The listing builds one solid part. Answer for the finished solid, in the listing's coordinates (mm). Face numbers are marked on the shaded views. A direction names the side the tool comes from. Coordinates: 2 decimals unless noted, no trailing zeros. Order: outer loops, then holes, each group sorted by start corner. A loop starts at its lowest first (then second) coordinate and runs counter-clockwise, first axis right, second up. Notation, with made-up numbers: (-18.5, 22.25) -> (35.5, 22.25) arc R24 cw to (35.5, 61.25) -> close; hole circle Ø3 at (73, 64). An arc over 180 degrees is marked (long way). Return JSON: item names as keys, results as strings.
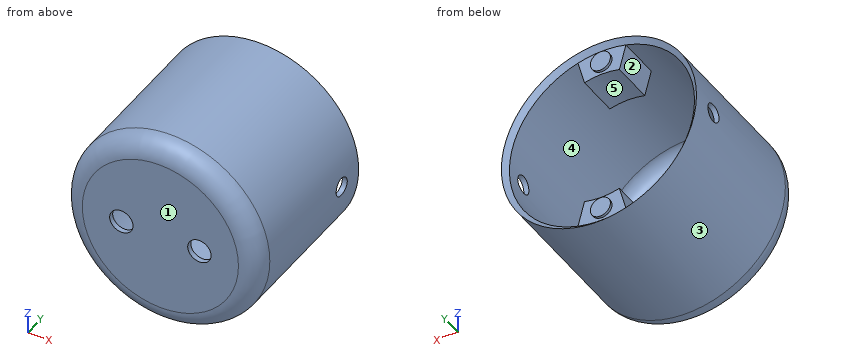
Autodesk Inventor part; units mm, degrees
ref_plane "Plano de trabajo1" through (-8, 0, 0) normal (1, 0, 0) x (0, 1, 0)
ref_plane "XZ Plane" through (0, 0, 0) normal (0, 1, 0) x (-1, 0, 0)
ref_plane "XY Plane" through (0, 0, 0) normal (0, 0, 1) x (1, 0, 0)
sketch "Boceto1" plane through (0, 0, 0) normal (0, 0, 1) x (1, 0, 0)
  line L0 (0, 0) -> (-4.6715, 0)
  line L1 (-5.8393, 9.9269) -> (-5.8393, 1.1679)
  line L2 (-5.5393, 9.6269) -> (-5.5393, 1.1679)
  arc A0 (-5.8393, 1.1679) -> (-4.6715, 0) centre (-4.6715, 1.1679) ccw
  arc A1 (-5.5393, 1.1679) -> (-4.6715, 0.3) centre (-4.6715, 1.1679) ccw
  line L3 (0, 0) -> (-4.6715, 0)
  line L4 (0, 0.3) -> (-4.6715, 0.3)
  line L5 (0, 0.3) -> (0, 0)
  line L6 (-5.8393, 9.9269) -> (-5.5393, 9.6269)
revolve "Revolución1" add sketch "Boceto1" angle 360 about axis through (0, 0.3, 0) along (0, -1, 0)
sketch "Boceto2" plane through (0, 0, 0) normal (1, 0, 0) x (0, 1, 0)
  line L0 (9.6269, 5.5393) -> (1.1679, 5.5393)
  line L1 (9.6269, -5.5393) -> (1.1679, -5.5393)
  line L2 (9.6269, 5.5393) -> (9.6269, 4.0393)
  line L3 (9.6269, -5.5393) -> (9.6269, 5.5393)
  line L4 (9.6269, 4.0393) -> (7.1269, 4.0393)
  line L5 (7.1269, 4.0393) -> (7.1269, 5.5393)
  line L6 (9.6269, 5.5393) -> (7.1269, 5.5393)
  line L7 (9.6269, 0) -> (13.8106, 0)
  line L8 (9.6269, -5.5393) -> (9.6269, -4.0393)
  line L9 (9.6269, -4.0393) -> (7.1269, -4.0393)
  line L10 (7.1269, -4.0393) -> (7.1269, -5.5393)
  point P0 (0, 0)
  dimension "d1" = 1.5
  dimension "d2" = 2.5
  dimension "d3" = 1.5
  dimension "d4" = 2.5
revolve "Revolución2" add sketch "Boceto2" angle 30 mid plane about axis through (0, 9.6269, 0) along (0, 1, 0)
sketch "Boceto3" plane through (0, 9.6269, 0) normal (0, 1, 0) x (1, 0, 0)
  line L0 (-1.0455, -3.9017) -> (-1.4337, -5.3506)
  arc A0 (-1.4337, -5.3506) -> (1.4337, -5.3506) centre (0, 0) ccw
  line L1 (1.0455, -3.9017) -> (1.4337, -5.3506)
  arc A1 (-1.0455, -3.9017) -> (1.0455, -3.9017) centre (0, 0) ccw
  line L2 (1.4337, 5.3506) -> (1.0455, 3.9017)
  arc A2 (1.4337, 5.3506) -> (-1.4337, 5.3506) centre (0, 0) ccw
  line L3 (-1.0455, 3.9017) -> (-1.4337, 5.3506)
  arc A3 (1.0455, 3.9017) -> (-1.0455, 3.9017) centre (0, 0) ccw
  circle A4 centre (0, 4.7895) radius 0.6
  circle A5 centre (0, -4.7895) radius 0.6
  dimension "d9" = 1.2
  dimension "d10" = 1.2
extrude "Extrusión1" add sketch "Boceto3" along normal blind 0.155 contours A4 | A5
ref_plane "Plano de trabajo1" through (-8, 0, 0) normal (1, 0, 0) x (0, 1, 0)
sketch "Boceto6" plane through (-8, 0, 0) normal (1, 0, 0) x (0, 1, 0)
  line L0 (1.1679, -5.8393) -> (1.1679, 5.8393)
  line L1 (9.9269, -5.8393) -> (9.9269, 5.8393)
  line L2 (0, -4.6715) -> (0, 4.6715)
  line L3 (1.1679, -5.8393) -> (1.1679, 5.8393)
  circle A0 centre (8.2551, 0) radius 0.55
  point P0 (0, 0)
extrude "Extrusión2" cut sketch "Boceto6" along normal blind 16
sketch "Boceto7" plane through (0, 0, 0) normal (0, -1, 0) x (1, 0, 0)
  circle A0 centre (-2.3358, 0) radius 0.7
  circle A1 centre (2.3358, 0) radius 0.7
  point P0 (0, 0)
  dimension "d17" = 1.4
  dimension "d18" = 1.4
extrude "Extrusión3" cut sketch "Boceto7" against normal blind 3
properties part number "cuerpo"
Item 1: The part is cut by section A-A on z = 0. Determine the outline of the cut face in (x, y).
Answer list:
{"outline": "(-5.84, 1.17) arc R1.17 ccw to (-4.67, 0) -> (-3.04, 0) -> (-3.04, 0.3) -> (-4.67, 0.3) arc R0.87 cw to (-5.54, 1.17) -> (-5.54, 7.71) -> (-5.84, 7.71) -> close; (-5.84, 8.81) -> (-5.54, 8.81) -> (-5.54, 9.63) -> (-5.84, 9.93) -> close; (-1.64, 0) -> (1.64, 0) -> (1.64, 0.3) -> (-1.64, 0.3) -> close; (3.04, 0) -> (4.67, 0) arc R1.17 ccw to (5.84, 1.17) -> (5.84, 7.71) -> (5.54, 7.71) -> (5.54, 1.17) arc R0.87 cw to (4.67, 0.3) -> (3.04, 0.3) -> close; (5.54, 8.81) -> (5.84, 8.81) -> (5.84, 9.93) -> (5.54, 9.63) -> close"}
Item 2: Find the intervals of material crossed by probe 1 along X at (y, z) = (8, 4.25); probe 2 along Y at (x, z) = (1.25, 1.25); probe 3 along X at (y, z) = (8.25, -3), in increasing order.
Answer list:
{"probe 1": "-4 to -3.55, -1.14 to 1.14, 3.55 to 4", "probe 2": "0 to 0.3", "probe 3": "-5.01 to -4.66, 4.66 to 5.01"}
Item 3: The part is cut by section B-B on y = 4.75. Determine the outline of the cut face in (x, z).
Answer list:
{"outline": "circle Ø11.68 at (0, 0); hole circle Ø11.08 at (0, 0)"}
Item 4: The part is cut by section C-C on x = 0. Determine the outline of the cut face in (y, z).
Answer list:
{"outline": "(0, -4.67) arc R1.17 ccw to (1.17, -5.84) -> (9.93, -5.84) -> (9.63, -5.54) -> (9.63, -5.39) -> (9.78, -5.39) -> (9.78, -4.19) -> (9.63, -4.19) -> (9.63, -4.04) -> (7.13, -4.04) -> (7.13, -5.54) -> (1.17, -5.54) arc R0.87 cw to (0.3, -4.67) -> (0.3, 4.67) arc R0.87 cw to (1.17, 5.54) -> (7.13, 5.54) -> (7.13, 4.04) -> (9.63, 4.04) -> (9.63, 4.19) -> (9.78, 4.19) -> (9.78, 5.39) -> (9.63, 5.39) -> (9.63, 5.54) -> (9.93, 5.84) -> (1.17, 5.84) arc R1.17 ccw to (0, 4.67) -> close"}
Item 5: Flat-ended cylindrical pins translate along their axes: pin 1 (2 mm diameter, centred on x = -3, z = -3, fed in from +Y); pin 2 (0.8 mm diameter, centred on x = 0.5, z = 4.5, fed in from +Y); pin 3 (5 mm diameter, centred on x = 3, y = 5, fed in from -Z). Find the tip coordinate at first contact, or state that the pin passes through.
Answer list:
{"pin 1": "y = 0.51", "pin 2": "y = 9.78", "pin 3": "z = -5.82"}
Item 6: Determine the mould class of the marked faces 1, 2 and 3 for opening direction Z: pulls with the +Z half, pulls with the -Z half, needs draft (parallel to the pull), parting line crosses it, or undercut.
Answer list:
{"face 1": "needs draft", "face 2": "undercut", "face 3": "parting line crosses it"}
Item 7: Which of the six approach directions +Z, -Z, +X, -X, +Y, -Y give full straight-line access (tool end or side, diameter ignored) to the marked faces 4 and 5?
Answer list:
{"face 4": "none", "face 5": "+Y"}
